Work out the finished part from the listing and answer in its coordinate system (mm). Give positions to 0.01 mm unless a question says otherwise; leave off trailing zeros. Loops run counter-clockwise (first coordinate to the right, second up) from the corner with the lowest first, then second, coordinate; pieces in that order, holes last. Notation, with made-up numbers: (30, 59.5) -> (37, 59.5) arc R12 ccw to (37, 80.5) -> close; hole circle Ø10 at (31.25, 38). An arc over 180 degrees is marked (long way). Answer as CSV lines item,"result". Start each with the question number.
1. Flat-ended cylindrical pins translate along their axes: pin 1 Ø3 at (x, z) = (45.5, -2) entering from +Y; pin 2 Ø0.6 at (x, y) = (32, 1.5) entering from +Z; pin 3 Ø1.5 at (y, z) = (1.5, -2) entering from -X. Find the tip coordinate at first contact, or state that the pin passes through.
2. Find the intervals of material crossed by line 1 along Y through (x, z) = (52.5, 7.75); line 2 along Z through (x, y) = (8.5, 1.2); line 3 along Z through (x, y) = (27, 1.95), in increasing order.
3. Find section B-B, the plane x = 46. Give the vertices of the cut face in (y, z).
4. Find section A-A, the plane z = -1.25. Count the separate pieces of the cut face and the enclosed holes in it, and give its area (3 significant figures).
5. Determine the mould class of faces 1 (the face through (14, 1, 3.5)), 2 (the face through (49.8, 1.3, -3.2)), 3 (the face through (19, 1, 3.5)) for opening direction Y: +Y half, -Y half, draft (parallel to the pull), parting line (faces both ways), or undercut.
from build123d import *

# Parameters (mm, degrees)
SKETCH_1_W             = 56.38
SKETCH_1_H             = 2.5
EXTRUDE_1_DEPTH        = 8.5
SKETCH_2_W             = 1.210634416
SKETCH_2_H             = 1.563190286
CUT_EXTRUDE_1_DEPTH    = 5
PATTERN_LINEAR_1_COUNT = 12
PATTERN_LINEAR_1_PITCH = 2.54
PATTERN_LINEAR_2_COUNT = 11
PATTERN_LINEAR_2_PITCH = 2.54
SKETCH_3_R             = 0.45
EXTRUDE_2_DEPTH        = 3.2
PATTERN_LINEAR_3_COUNT = 22
PATTERN_LINEAR_3_PITCH = 2.54


with BuildPart() as part:
    # 草图1 → 凸台-拉伸1 (new body)
    with BuildSketch(Plane.XY):
        with Locations((28.19, 1.25)):
            Rectangle(SKETCH_1_W, SKETCH_1_H)
    extrude(amount=EXTRUDE_1_DEPTH)

    # 草图2 → 切除-拉伸1 (cut)
    with BuildSketch(Plane.XY.offset(8.5)):
        with Locations((26.92, 1.25)):
            Rectangle(SKETCH_2_W, SKETCH_2_H)
    cut_extrude_1 = extrude(amount=-CUT_EXTRUDE_1_DEPTH, mode=Mode.SUBTRACT)

    # 阵列(线性)1: 切除-拉伸1 ×12
    with Locations(*[(i * PATTERN_LINEAR_1_PITCH, 0, 0) for i in range(1, PATTERN_LINEAR_1_COUNT)]):
        add(cut_extrude_1, mode=Mode.SUBTRACT)

    # 阵列(线性)2: 切除-拉伸1 ×11
    with Locations(*[(-i * PATTERN_LINEAR_2_PITCH, 0, 0) for i in range(1, PATTERN_LINEAR_2_COUNT)]):
        add(cut_extrude_1, mode=Mode.SUBTRACT)

    # 草图3 → 凸台-拉伸2 (add)
    with BuildSketch(Plane(origin=(0, 0, 0), x_dir=(-1, 0, 0), z_dir=(0, 0, -1))):
        with Locations((-54.86, 1.25)):
            Circle(SKETCH_3_R)
    extrude_2 = extrude(amount=EXTRUDE_2_DEPTH)

    # 阵列(线性)3: 凸台-拉伸2 ×22
    with Locations(*[(-i * PATTERN_LINEAR_3_PITCH, 0, 0) for i in range(1, PATTERN_LINEAR_3_COUNT)]):
        add(extrude_2)


solid = part.part
Resolved:
1,pin 1,"stops at y = 1.7"
1,pin 2,"stops at z = 3.5"
1,pin 3,"stops at x = 1.07"
2,line 1,"y = 0 to 0.47, 2.03 to 2.5"
2,line 2,"z = 0 to 8.5"
2,line 3,"z = 0 to 3.5"
3,outline,"(0, 0) -> (2.5, 0) -> (2.5, 8.5) -> (0, 8.5) -> close"
4,separate pieces,"22"
4,enclosed holes,"0"
4,area,"14.0 mm^2"
5,face 1,"undercut"
5,face 2,"draft"
5,face 3,"undercut"
